Model file for the job. Use its own axes, mm. A direction names the side the tool comes from. Coordinates: 2 decimals unless noted, no trailing zeros. Write each loop counter-clockwise with the first axis right and the second up, starting at its lowest first coordinate (ties: lowest second). Pieces come first, ordered by that corner, then holes. Notation, with made-up numbers: M 19,-35 L 51,-35 A5 ccw 51,-29 Z; hole C 18,-1 d9. An arc over 180 degrees is marked long. Put each result on its own line as item: value. Start each with the question number.
Q1. Pull direction Y, two halves, no side cores. Call faces 1 (the cylindrical face through (-0.15, -12.1, 2.54)), 2 (the cylindrical face through (-12.1, 7.11, 2.54)), 3 (the flat face through (0, 12.7, 0)), 4 (the cylindrical face through (-4.84, -0.07, 2.54)): pulls with the +Y half, pulls with the -Y half, needs draft (parallel to the pull), parting line crosses it, or undercut.
Q2. Drill centre lines: line 1 along Y through (x, z) = (0, 0.7); line 2 along Y through (x, z) = (-6.5, 0.1); line 3 along Z through (x, y) = (-7, -8) (3 decimals). Where is each one in solid material? Low to high.
Q3. Drop flat-ended pins along their axis: pin 1 (1.1 mm diameter, centred on y = 11.5, z = -1.5, fed in from -X) (3 decimals); pin 2 (7.5 mm diameter, centred on x = 0.5, y = -3, fed in from -Z); pin 3 (0.9 mm diameter, centred on y = 0.5, z = 0.5, fed in from -X). Give the stop position or say it passes through.
Q4. Cut at B-B (y = 0). Write the cut outline in (x, z) (3 decimals).
Q5. Cut at D-D (x = 9.5). Write the cut outline in (y, z) (3 decimals), then the cut area to 3 significant figures.
Q6. Cut at C-C (z = 1.8). Write the cut outline in (x, y).
Q7. Cut at A-A (x = -6.75). Write the cut outline in (y, z) (3 decimals), then the cut area to 3 significant figures.
Q8. Which spindle directions (+Z, -Z, +X, -X, +Y, -Y) get a long thin tool onto all of the face, cutting with end or side? Do faces 5 (the flat face through (12.7, 0.1, 0.5)), 6 (the cylindrical face through (-8.08, 4.12, 2.54)), 7 (the flat face through (-5.442, -0.2, 0.5)), 8 (the flat face through (3.175, 12, -1)). Say none if no direction does.
```python
from build123d import *

# Parameters (mm, degrees)
BOSS_EXTRUDE1_DEPTH = 3.175
FILLET1_R           = 2.1082
CUT_EXTRUDE1_REACH  = 5.175
SKETCH2_R           = 3.2639
SKETCH3_W           = 6.35
SKETCH3_H           = 2.1082
BOSS_EXTRUDE2_DEPTH = 2.1082


with BuildPart() as part:
    # Sketch1 → Boss-Extrude1 (new body)
    with BuildSketch(Plane.XY):
        Polygon((-12.7, 12.7), (12.7, 12.7), (12.7, -12.7), (-12.7, -12.7), (-12.7, -3.822069256), (-5.441576375, -3.822069256), (-5.441576375, 3.520801512), (-12.7, 3.520801512), align=None)
    extrude(amount=BOSS_EXTRUDE1_DEPTH)

    # Fillet1
    fillet1_edges = [part.edges().sort_by_distance(p)[0] for p in [
        (-5.441576375, -0.150633872, 3.175),
        (-9.070788187, -3.822069256, 3.175),
        (-12.7, 12.7, 1.5875),
        (12.7, 12.7, 1.5875),
        (12.7, -12.7, 1.5875),
        (-12.7, -12.7, 1.5875),
        (-12.7, -8.261034628, 3.175),
        (0, -12.7, 3.175),
        (12.7, 0, 3.175),
        (0, 12.7, 3.175),
        (-12.7, 8.110400756, 3.175),
        (-9.070788187, 3.520801512, 3.175),
    ]]
    fillet(fillet1_edges, radius=FILLET1_R)

    # Sketch2 → Cut-Extrude1 (cut, up to next)
    with BuildSketch(Plane.XY.offset(3.175), mode=Mode.PRIVATE) as cut_extrude1_sk1:
        Circle(SKETCH2_R)
    cut_extrude1_tool1 = extrude(cut_extrude1_sk1.sketch, amount=-CUT_EXTRUDE1_REACH, mode=Mode.PRIVATE) & part.part
    add(cut_extrude1_tool1.solids().sort_by_distance((0, 0, 3.175))[0], mode=Mode.SUBTRACT)

    # Sketch3 → Boss-Extrude2 (add)
    with BuildSketch(Plane(origin=(0, 0, 0), x_dir=(-1, 0, 0), z_dir=(0, 0, -1))):
        with Locations((0, 11.6459)):
            Rectangle(SKETCH3_W, SKETCH3_H)
    extrude(amount=BOSS_EXTRUDE2_DEPTH)


solid = part.part
```
Computed values:
1. face 1: pulls with the -Y half
1. face 2: needs draft
1. face 3: pulls with the +Y half
1. face 4: undercut
2. line 1: -12.7 to -3.26, 3.26 to 12.7
2. line 2: -12.7 to -3.82, 3.52 to 12.7
2. line 3: 0 to 3.175
3. pin 1: x = -3.175
3. pin 2: z = 0
3. pin 3: x = -5.44
4. outline: M -5.442,0 L -3.264,0 L -3.264,3.175 L -3.333,3.175 A2.108 ccw -5.442,1.067 Z; M 3.264,0 L 12.7,0 L 12.7,1.067 A2.108 ccw 10.592,3.175 L 3.264,3.175 Z
5. outline: M -12.7,0 L 12.7,0 L 12.7,1.067 A2.108 ccw 10.592,3.175 L -10.592,3.175 A2.108 ccw -12.7,1.067 Z
5. area: 78.7 mm2
6. outline: M -12.57,-10.59 A1.98 ccw -10.59,-12.57 L 10.59,-12.57 A1.98 ccw 12.57,-10.59 L 12.57,10.59 A1.98 ccw 10.59,12.57 L -10.59,12.57 A1.98 ccw -12.57,10.59 L -12.57,3.65 L -5.31,3.65 L -5.31,-3.95 L -12.57,-3.95 Z; hole C 0,0 d6.53
7. outline: M -12.7,0 L -3.822,0 L -3.822,1.067 A2.108 ccw -5.93,3.175 L -10.592,3.175 A2.108 ccw -12.7,1.067 Z; M 3.521,0 L 12.7,0 L 12.7,1.067 A2.108 ccw 10.592,3.175 L 5.629,3.175 A2.108 ccw 3.521,1.067 Z
7. area: 53.5 mm2
8. face 5: +Z, -Z, +X, +Y, -Y
8. face 6: +Z, -X
8. face 7: +Z, -Z, -X
8. face 8: -Z, +X, +Y, -Y
